```python
from build123d import *

# Parameters (mm, degrees)
SKETCH1_R             = 1.13
BOSS_EXTRUDE1_DEPTH   = 2.54
FILLET1_R             = 20
FILLET6_R             = 6.35
FILLET7_R             = 1
F_4_40_TAPPED_HOLE1_D = 2.2606


with BuildPart() as part:
    # Sketch1 → Boss-Extrude1 (new body)
    with BuildSketch(Plane(origin=(0, 0, 0), x_dir=(1, 0, 0), z_dir=(0, 1, 0))):
        with BuildLine():
            Line((11.225, 0), (0, 0))
            Line((0, 0), (0, -125))
            Line((0, -125), (127, -125))
            Line((127, -125), (127, 0))
            Line((127, 0), (115.775, 0))
            Line((115.775, 0), (115.775, -111))
            ThreePointArc((115.775, -111), (114.3, -112.475), (112.825, -111))
            Line((112.825, -111), (112.825, 0))
            Line((112.825, 0), (14.175, 0))
            Line((14.175, 0), (14.175, -111))
            ThreePointArc((14.175, -111), (12.7, -112.475), (11.225, -111))
            Line((11.225, -111), (11.225, 0))
        make_face()
        with BuildLine():
            ThreePointArc((71, -97.5), (63.5, -105), (56, -97.5))
            Line((56, -97.5), (56, -82.5))
            ThreePointArc((56, -82.5), (63.5, -75), (71, -82.5))
            Line((71, -82.5), (71, -97.5))
        make_face(mode=Mode.SUBTRACT)
        with Locations(Location((106.5, -4.5, 0), (0, 0, 270))):
            Circle(SKETCH1_R, mode=Mode.SUBTRACT)
        with Locations(Location((20.5, -90.5, 0), (0, 0, 270))):
            Circle(SKETCH1_R, mode=Mode.SUBTRACT)
        with Locations(Location((106.5, -90.5, 0), (0, 0, 270))):
            Circle(SKETCH1_R, mode=Mode.SUBTRACT)
        with Locations(Location((20.5, -4.5, 0), (0, 0, 270))):
            Circle(SKETCH1_R, mode=Mode.SUBTRACT)
    extrude(amount=BOSS_EXTRUDE1_DEPTH)

    # Fillet1
    # the kernel refuses this fillet: 20 mm, written as the material it takes off along each edge
    with BuildSketch(Plane(origin=(0, -44.930458419, 0), x_dir=(1, 0, 0), z_dir=(0, 1, 0))) as fillet1_piece_1:
        with BuildLine():
            CenterArc((20, -17.972183368), FILLET1_R, 116.024153389, 63.975846611)
            Line((0, -17.972183368), (-0.4, -17.972183368))
            Line((-0.4, -17.972183368), (-0.4, 0))
            Line((-0.4, 0), (0, 0.4))
            ThreePointArc((0, 0.4), (5.6125, 0.4), (11.0495, 0.359443667))
            Line((11.0495, 0.359443667), (11.225, 0))
        make_face()
    extrude(amount=92.400916838, mode=Mode.SUBTRACT)
    with BuildSketch(Plane(origin=(127, -44.930458419, 0), x_dir=(0, 0, 1), z_dir=(0, 1, 0))) as fillet1_piece_2:
        with BuildLine():
            CenterArc((17.972183368, -20), FILLET1_R, 90, 63.975846611)
            Line((0, -11.225), (-0.359443667, -11.0495))
            ThreePointArc((-0.359443667, -11.0495), (-0.4, -5.6125), (-0.4, 0))
            Line((-0.4, 0), (0, 0.4))
            Line((0, 0.4), (17.972183368, 0.4))
            Line((17.972183368, 0.4), (17.972183368, 0))
        make_face()
    extrude(amount=92.400916838, mode=Mode.SUBTRACT)
    with BuildSketch(Plane(origin=(127, -50, 125), x_dir=(-1, 0, 0), z_dir=(0, 1, 0)), Plane(origin=(0, -50, 125), x_dir=(0, 0, -1), z_dir=(0, 1, 0))) as fillet1_piece_3:
        with BuildLine():
            CenterArc((FILLET1_R, -FILLET1_R), FILLET1_R, 90, 90)
            Line((0, -FILLET1_R), (-FILLET1_R * 0.02, -FILLET1_R))
            Line((-FILLET1_R * 0.02, -FILLET1_R), (-FILLET1_R * 0.02, FILLET1_R * 0.02))
            Line((-FILLET1_R * 0.02, FILLET1_R * 0.02), (FILLET1_R, FILLET1_R * 0.02))
            Line((FILLET1_R, FILLET1_R * 0.02), (FILLET1_R, 0))
        make_face()
    extrude(amount=102.54, mode=Mode.SUBTRACT)

    # Fillet6
    fillet6_edges = [part.edges().sort_by_distance(p)[0] for p in [
        (112.825, 1.27, 0),
        (14.175, 1.27, 0),
    ]]
    fillet(fillet6_edges, radius=FILLET6_R)

    # Fillet7
    fillet7_edges = [part.edges().sort_by_distance(p)[0] for p in [
        (115.775, 1.27, 0),
        (11.225, 1.27, 0),
    ]]
    fillet(fillet7_edges, radius=FILLET7_R)

    # #4-40 Tapped Hole1 (through all)
    with Locations(Plane(origin=(106.5, 2.54, 4.5), x_dir=(0, 0, 1), z_dir=(0, 1, 0))):
        with Locations((0, 0), (0, -86), (86, 0), (86, -86)):
            Hole(F_4_40_TAPPED_HOLE1_D / 2)


solid = part.part
```
Here's how the part is built. I have some questions about the finished solid (model axes, mm). A direction names the side the tool comes from. Coordinates: 2 decimals unless noted, no trailing zeros. Write each loop counter-clockwise with the first axis right and the second up, starting at its lowest first coordinate (ties: lowest second). Pieces come first, ordered by that corner, then holes. Notation, with made-up numbers: (43.5, 53) -> (83.5, 53) arc R9 cw to (83.5, 67) -> close; hole circle Ø7 at (-36.75, -8). An arc over 180 degrees is marked (long way). Use a Markdown table: item, result. Add a question column.
(1) If we section it at D-D, the plane z = 85.5: Write out the boundary of the cut face in (x, y) (3 decimals), and give its area (3 significant figures).
(2) We'd pull the mould along Z, two halves only. Please class faces 4 (the cylindrical face through (63.34, 1.25, 75)), 5 (the flat face through (63, 2.54, 62)), 6 (the cylindrical face through (2.67, 1.25, 7.99)): +Z half, -Z half, draft (parallel to the pull), parting line (faces both ways), or undercut.
(3) If we section it at A-A, the plane x = 63.5: Write out the boundary of the cut face in (y, z), and give its area (3 significant figures).
(4) I'm going to push flat-ended pins straight in: P1, Ø2, axis at x = 20.5, z = 4.5, coming from the -Y side; P2, Ø4, axis at x = 94.5, z = 92, coming from the -Y side. Where does each tip first touch, or does it pass through?
(5) If we section it at C-C, the plane y = 1.5: Write out the boundary of the cut face in (x, z) (3 decimals).
(6) For faces 1 (the cylindrical face through (124.474, 1.252, 8.244)), 2 (the cylindrical face through (63.66, 1.25, 105)), 3 (the cylindrical face through (15.986, 1.288, 1.91)), which set-ups out of +Z, -Z, +X, -X, +Y, -Y let a thin tool reach every point of the face, with its end or its side?
(7) Please list where these lines run through material, in increasing order: line 1 (X direction, y = 1.8, z = 57) (3 decimals); line 2 (Z direction, x = 106.5, y = 0.5); line 3 (X direction, y = 0.25, z = 101) (3 decimals).
(8) If we section it at B-B, the plane z = 53: Write out the boundary of the cut face in (x, y) (3 decimals).
Outcome:
| question | item | result |
|---|---|---|
| 1 | outline | (0, 0) -> (11.225, 0) -> (11.225, 2.54) -> (0, 2.54) -> close; (14.175, 0) -> (56, 0) -> (56, 2.54) -> (14.175, 2.54) -> close; (71, 0) -> (112.825, 0) -> (112.825, 2.54) -> (71, 2.54) -> close; (115.775, 0) -> (127, 0) -> (127, 2.54) -> (115.775, 2.54) -> close |
| 1 | area | 269 mm^2 |
| 2 | face 4 | undercut |
| 2 | face 5 | draft |
| 2 | face 6 | -Z half |
| 3 | outline | (0, 0) -> (2.54, 0) -> (2.54, 75) -> (0, 75) -> close; (0, 105) -> (2.54, 105) -> (2.54, 125) -> (0, 125) -> close |
| 3 | area | 241 mm^2 |
| 4 | P1 | passes through |
| 4 | P2 | stops at y = 0 |
| 5 | outline | (0, 17.972) arc R20 ccw to (9.711, 0.822) arc R1 ccw to (11.225, 1.68) -> (11.225, 111) arc R1.475 cw to (14.175, 111) -> (14.175, 6.35) arc R6.35 ccw to (20.525, 0) -> (106.475, 0) arc R6.35 ccw to (112.825, 6.35) -> (112.825, 111) arc R1.475 cw to (115.775, 111) -> (115.775, 1.68) arc R1 ccw to (117.289, 0.822) arc R20 ccw to (127, 17.972) -> (127, 105) arc R20 ccw to (107, 125) -> (20, 125) arc R20 ccw to (0, 105) -> close; hole circle Ø2.261 at (20.5, 4.5); hole circle Ø2.261 at (20.5, 90.5); hole (56, 82.5) arc R7.5 ccw to (71, 82.5) -> (71, 97.5) arc R7.5 ccw to (56, 97.5) -> close; hole circle Ø2.261 at (106.5, 4.5); hole circle Ø2.261 at (106.5, 90.5) |
| 6 | face 1 | -Z, +X, +Y, -Y |
| 6 | face 2 | +Y, -Y |
| 6 | face 3 | -Z, +Y, -Y |
| 7 | line 1 | x = 0 to 11.225, 14.175 to 112.825, 115.775 to 127 |
| 7 | line 2 | z = 0 to 3.37, 5.63 to 89.37, 91.63 to 125 |
| 7 | line 3 | x = 0 to 11.225, 14.175 to 56.867, 70.133 to 112.825, 115.775 to 127 |
| 8 | outline | (0, 0) -> (11.225, 0) -> (11.225, 2.54) -> (0, 2.54) -> close; (14.175, 0) -> (112.825, 0) -> (112.825, 2.54) -> (14.175, 2.54) -> close; (115.775, 0) -> (127, 0) -> (127, 2.54) -> (115.775, 2.54) -> close |
